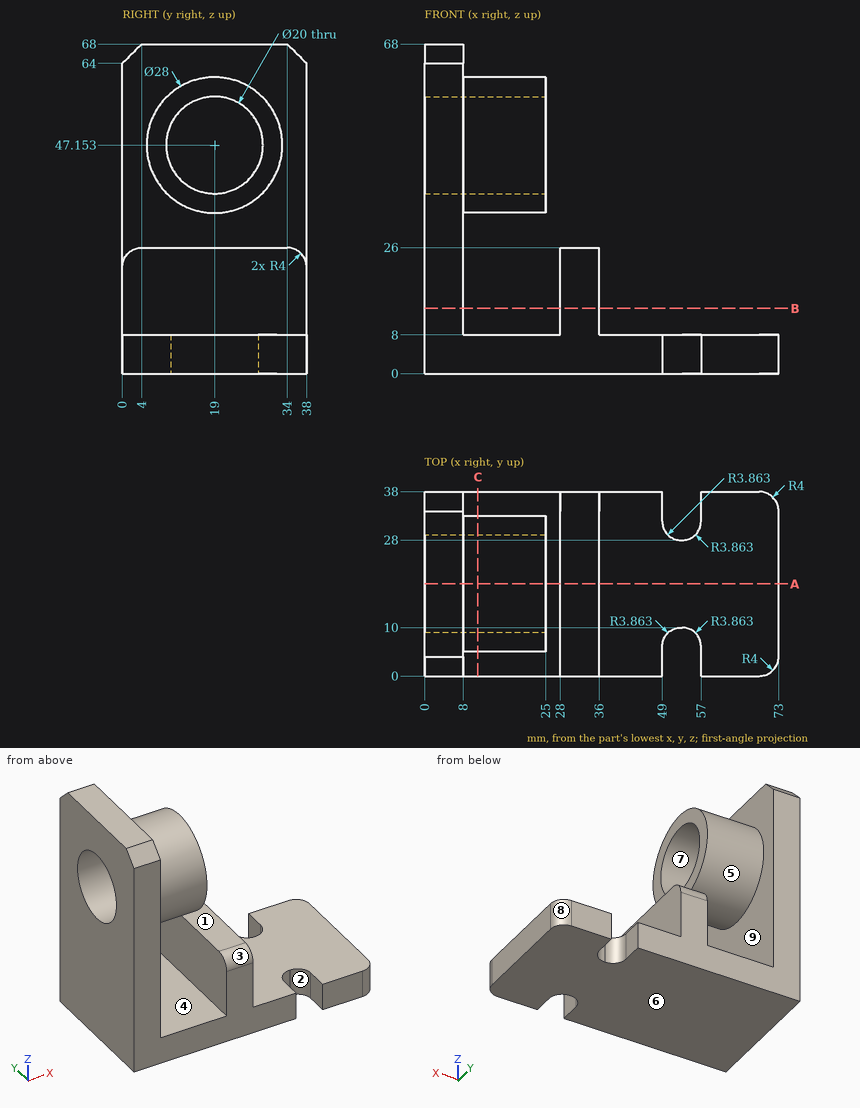
Answer from the drawing. Dimensions are ordinates in mm from the lowest x, y and z of the part. A direction names the side the tool comes from. Coordinates: 2 decimals unless noted, no trailing zeros. Order: outer loops, then holes, each group sorted by start corner. A loop starts at its lowest first (then second) coordinate and runs counter-clockwise, first axis right, second up. Notation, with made-up numbers: (19.5, 83) -> (27.5, 83) arc R28 cw to (27.5, 115) -> close; hole circle Ø10 at (-27.75, -1). An arc over 180 degrees is marked (long way). Answer as a JSON object with one key per item and string values.
1) Consider line 1 along Z through (x, y) = (18, 19); line 2 along X through (y, z) = (3.5, 15); line 3 along Z through (x, y) = (12, 22). Determine where each line is inside the solid, lowest interval first. Write a range as from..to.
Model answer:
{"line 1": "z = 0..8, 33.15..37.15, 57.15..61.15", "line 2": "x = 0..8, 28..36", "line 3": "z = 0..8, 33.48..37.61, 56.69..60.83"}
2) A cutting plane is placed at C-C, the plane x = 11. Determine the outline of the cut face in (y, z).
Model answer:
{"outline": "(0, 0) -> (38, 0) -> (38, 8) -> (0, 8) -> close; circle Ø28 at (19, 47.15); hole circle Ø20 at (19, 47.15)"}
3) A cutting plane is placed at B-B, the plane z = 13.5. Determine the outline of the cut face in (x, y), plus the area to 3 significant figures.
Model answer:
{"outline": "(0, 0) -> (8, 0) -> (8, 38) -> (0, 38) -> close; (28, 0) -> (36, 0) -> (36, 38) -> (28, 38) -> close", "area": "608 mm²"}
4) A cutting plane is placed at A-A, the plane y = 19. Determine the outline of the cut face in (x, z).
Model answer:
{"outline": "(0, 0) -> (73, 0) -> (73, 8) -> (36, 8) -> (36, 26) -> (28, 26) -> (28, 8) -> (8, 8) -> (8, 33.15) -> (25, 33.15) -> (25, 37.15) -> (0, 37.15) -> close; (0, 57.15) -> (25, 57.15) -> (25, 61.15) -> (8, 61.15) -> (8, 68) -> (0, 68) -> close"}
5) The mould has two halves that part along Z. Classify the marked faces 6, 7, 8 and 9: released by +Z, released by -Z, zero draft, split by the parting line, or undercut.
Model answer:
{"face 6": "released by -Z", "face 7": "undercut", "face 8": "zero draft", "face 9": "undercut"}
6) Each of these flat-tipped pins is pushed along its axis until it touches: pin 1 (2.5 mm diameter, centred on x = 33.5, y = 17, fed in from +Z); pin 2 (8 mm diameter, centred on x = 62.5, y = 13, fed in from +Z); pin 3 (8 mm diameter, centred on x = 13, z = 26.5, fed in from +Y); pin 4 (5 mm diameter, centred on x = 18.5, y = 19.5, fed in from +Z). Where does it stop, or does it pass through?
Model answer:
{"pin 1": "stops at z = 26", "pin 2": "stops at z = 8", "pin 3": "passes through", "pin 4": "stops at z = 61.15"}
7) A tool of negligible diameter and unlimited length cuts with its end or side. For the marked faces 1, 2, 3, 4 and 5, from which of +Z, -Z, +X, -X, +Y, -Y can it reach the whole face along a straight path? Write none if from no direction.
Model answer:
{"face 1": "+Z, +X, +Y, -Y", "face 2": "+Z, -Z, -Y", "face 3": "+Z, +X, -Y", "face 4": "+Y, -Y", "face 5": "+X"}
